Build history of the part. All positions in model axes, mm. Coordinates: 2 decimals unless noted, no trailing zeros. Order: outer loops, then holes, each group sorted by start corner. A loop starts at its lowest first (then second) coordinate and runs counter-clockwise, first axis right, second up. Notation, with made-up numbers: (-13.5, 65.25) - (-3.5, 65.25) arc R15 ccw to (-3.5, 69.25) - close; hole circle Ø4 at (81, 43.25). An arc over 180 degrees is marked (long way). Return JSON: item names as keys, results as strings.
Solid Edge part; units mm, degrees
sketch "Sketch1" plane through (0, 0, 0) normal (0, 0, 1) x (1, 0, 0)
  circle A0 centre (35.475, -40) radius 1.65
  circle A1 centre (16.425, -40) radius 1.65
  line L0 (11.95, -46) -> (39.95, -46)
  line L1 (39.95, -27) -> (39.95, -46)
  line L2 (11.95, -27) -> (39.95, -27)
  line L3 (11.95, -46) -> (11.95, -27)
extrude "Protrusion1" add sketch "Sketch1" against normal blind 0.8
properties material "ABS Plastic, high impact"
1. Probe L1, parallel to Y at x = 35.5, z = -0.4; L2, parallel to X at y = -41.25, z = -0.7; L3, parallel to Y at x = 17.5, z = -0.65. List the from-to ranges inside material, lowest first.
Check values:
{"L1": "-46 to -41.65, -38.35 to -27", "L2": "11.95 to 15.35, 17.5 to 34.4, 36.55 to 39.95", "L3": "-46 to -41.25, -38.75 to -27"}
2. Cut at B-B on z = -0.65. Give the cut face in (x, y) (3 decimals), plus the area to 3 significant figures.
Check values:
{"outline": "(11.95, -46) - (39.95, -46) - (39.95, -27) - (11.95, -27) - close; hole circle Ø3.3 at (16.425, -40); hole circle Ø3.3 at (35.475, -40)", "area": "515 mm²"}
3. Mould opens along X. For faces 1 (the cylindrical face through (36.362, -38.609, -0.394)), 2 (the cylindrical face through (15.209, -38.885, -0.394)), 3 (the flat face through (26, -36, -0.8)) say: pulls with the +X half, pulls with the -X half, needs draft (parallel to the pull), parting line crosses it, or undercut.
Check values:
{"face 1": "undercut", "face 2": "undercut", "face 3": "needs draft"}
4. Cut at D-D on x = 34.5. Give the cut face in (y, z), plus the area to 3 significant figures.
Check values:
{"outline": "(-46, -0.8) - (-41.33, -0.8) - (-41.33, 0) - (-46, 0) - close; (-38.67, -0.8) - (-27, -0.8) - (-27, 0) - (-38.67, 0) - close", "area": "13.1 mm²"}
5. Cut at A-A on y = -40. Give the cut face in (x, z) (3 decimals).
Check values:
{"outline": "(11.95, -0.8) - (14.775, -0.8) - (14.775, 0) - (11.95, 0) - close; (18.075, -0.8) - (33.825, -0.8) - (33.825, 0) - (18.075, 0) - close; (37.125, -0.8) - (39.95, -0.8) - (39.95, 0) - (37.125, 0) - close"}
6. Cut at C-C on x = 17. Give the cut face in (y, z).
Check values:
{"outline": "(-46, -0.8) - (-41.55, -0.8) - (-41.55, 0) - (-46, 0) - close; (-38.45, -0.8) - (-27, -0.8) - (-27, 0) - (-38.45, 0) - close"}
7. Drop a flat-ended pin along its axis: pin 1 (2 mm diameter, centred on x = 35.475, y = -40, fed in from -Z). Give the stop position or say it passes through.
Check values:
{"pin 1": "through"}
